from build123d import *

# Parameters (mm, degrees)
SKETCH_1_W               = 39
SKETCH_1_H               = 49
EXTRUDE_1_DEPTH          = 25
SKETCH_3_W               = 29
SKETCH_3_H               = 45
CUT_EXTRUDE_1_DEPTH      = 25
SKETCH_5_W               = 39
SKETCH_5_H               = 5
CUT_EXTRUDE_3_DEPTH      = 1
CUT_EXTRUDE_3_DEPTH_BACK = 26
HOLE_WIZARD_M4_4_D       = 3.3
SKETCH_20_W              = 39
SKETCH_20_H              = 5.65
CUT_EXTRUDE_5_DEPTH      = 1
CUT_EXTRUDE_5_DEPTH_BACK = 26
SKETCH_7_R               = 2.025
CUT_EXTRUDE_7_DEPTH      = 10
FILLET_1_R               = 2
FILLET_2_R               = 1
SKETCH_21_R              = 1.525
CUT_EXTRUDE_8_DEPTH      = 10


with BuildPart() as part:
    # 草图1 → 凸台-拉伸1 (new body)
    with BuildSketch(Plane.XY):
        Rectangle(SKETCH_1_W, SKETCH_1_H)
    extrude(amount=EXTRUDE_1_DEPTH)

    # 草图3 → 切除-拉伸1 (cut)
    with BuildSketch(Plane.XY.offset(25)):
        with Locations((0, -2)):
            Rectangle(SKETCH_3_W, SKETCH_3_H)
    extrude(amount=-CUT_EXTRUDE_1_DEPTH, mode=Mode.SUBTRACT)

    # 草图5 → 切除-拉伸3 (cut, two sides)
    with BuildSketch(Plane.XY.offset(25)) as cut_extrude_3_sk:
        with Locations((0, -22)):
            Rectangle(SKETCH_5_W, SKETCH_5_H)
    extrude(amount=CUT_EXTRUDE_3_DEPTH, mode=Mode.SUBTRACT)
    extrude(cut_extrude_3_sk.sketch, amount=-CUT_EXTRUDE_3_DEPTH_BACK, mode=Mode.SUBTRACT)

    # M4 螺纹孔4 (through all)
    with Locations(Plane(origin=(-19.5, 8.65, 5), x_dir=(0, 0, -1), z_dir=(-1, 0, 0))):
        with Locations((0, 0), (-15, 0), (-15, 15), (0, 15)):
            Hole(HOLE_WIZARD_M4_4_D / 2)

    # 草图20 → 切除-拉伸5 (cut, two sides)
    with BuildSketch(Plane.XY.offset(25)) as cut_extrude_5_sk:
        with Locations((0, -16.675)):
            Rectangle(SKETCH_20_W, SKETCH_20_H)
    extrude(amount=CUT_EXTRUDE_5_DEPTH, mode=Mode.SUBTRACT)
    extrude(cut_extrude_5_sk.sketch, amount=-CUT_EXTRUDE_5_DEPTH_BACK, mode=Mode.SUBTRACT)

    # 草图7 → 切除-拉伸7 (cut)
    with BuildSketch(Plane.XZ.offset(-20.5)):
        with Locations((-8.5, 20)):
            Circle(SKETCH_7_R)
        with Locations((-8.5, 5)):
            Circle(SKETCH_7_R)
        with Locations((8.5, 5)):
            Circle(SKETCH_7_R)
        with Locations((8.5, 20)):
            Circle(SKETCH_7_R)
    extrude(amount=-CUT_EXTRUDE_7_DEPTH, mode=Mode.SUBTRACT)

    # 圆角1
    fillet_1_edges = [part.edges().sort_by_distance(p)[0] for p in [
        (-14.5, 20.5, 12.5),
        (14.5, 20.5, 12.5),
        (-19.5, 24.5, 12.5),
        (19.5, 24.5, 12.5),
    ]]
    fillet(fillet_1_edges, radius=FILLET_1_R)

    # 圆角2
    fillet_2_edges = [part.edges().sort_by_distance(p)[0] for p in [
        (14.5, -13.85, 12.5),
        (-14.5, -13.85, 12.5),
        (-19.5, -13.85, 12.5),
        (19.5, -13.85, 12.5),
    ]]
    fillet(fillet_2_edges, radius=FILLET_2_R)

    # 草图21 → 切除-拉伸8 (cut)
    with BuildSketch(Plane(origin=(0, 24.5, 0), x_dir=(1, 0, 0), z_dir=(0, 1, 0))):
        with Locations((0, -6.15)):
            Circle(SKETCH_21_R)
        with Locations((0, -18.85)):
            Circle(SKETCH_21_R)
    extrude(amount=-CUT_EXTRUDE_8_DEPTH, mode=Mode.SUBTRACT)


solid = part.part
Read the model definition and answer for the solid it produces. Units are mm, in the model's axes. A direction names the side the tool comes from. Coordinates: 2 decimals unless noted, no trailing zeros. Loops run counter-clockwise (first coordinate to the right, second up) from the corner with the lowest first, then second, coordinate; pieces in that order, holes last. Notation, with made-up numbers: (49.5, 53) -> (54.5, 53) arc R11 ccw to (54.5, 74) -> close; hole circle Ø2 at (-27, -16). An arc over 180 degrees is marked (long way). Write item = value, one per line. Start each with the question number.
1) The part is cut by section B-B, the plane x = -8.5. Determine the outline of the cut face in (y, z) (3 decimals).
2) The part is cut by section A-A, the plane y = 13.5. Determine the outline of the cut face in (x, z), plus the area to 3 significant figures.
3) For faces 3 (the face through (17.03, -5.35, 18.69)), 4 (the face through (-14.5, 3, 13)), determine the directions among +Z, -Z, +X, -X, +Y, -Y from which every point of the face is accessible in a straight line to the end or side of a thin tool.
4) The part is cut by section D-D, the plane z = 16.5. Determine the outline of the cut face in (x, y).
5) The mould has two halves that part along X. Classify faces 1 (the face through (-16.97, -5.35, 3.69)), 2 (the face through (-0.2, 22.53, 17.34)): pulls with the +X half, pulls with the -X half, needs draft (parallel to the pull), parting line crosses it, or undercut.
6) Find the intervals of material crossed by L1, parallel to Z at x = 17.65, y = -6.35; L2, parallel to Z at x = 0, y = 22 (3 decimals); L3, parallel to Y at x = 16.9, z = 20, in increasing order. Write a range as from..to.
7) Given P1, Ø5.5, axis at x = -8.5, z = 20, coming from the -Y side, flat-ended and moving along its own axis, determine where the tip first touches the part or whether it passes through.
8) The part is cut by section C-C, the plane y = -6.35. Determine the outline of the cut face in (x, z), plus the area to 3 significant figures.
Result:
q1.outline = (20.5, 0) -> (24.5, 0) -> (24.5, 2.975) -> (20.5, 2.975) -> close; (20.5, 7.025) -> (24.5, 7.025) -> (24.5, 17.975) -> (20.5, 17.975) -> close; (20.5, 22.025) -> (24.5, 22.025) -> (24.5, 25) -> (20.5, 25) -> close
q2.outline = (-19.5, 0) -> (-14.5, 0) -> (-14.5, 25) -> (-19.5, 25) -> close; (14.5, 0) -> (19.5, 0) -> (19.5, 25) -> (14.5, 25) -> close
q2.area = 250 mm²
q3.face_3 = +X, -X
q3.face_4 = +Z, -Z, -Y
q4.outline = (-19.5, -12.85) arc R1 ccw to (-18.5, -13.85) -> (-15.5, -13.85) arc R1 ccw to (-14.5, -12.85) -> (-14.5, 18.5) arc R2 cw to (-12.5, 20.5) -> (12.5, 20.5) arc R2 cw to (14.5, 18.5) -> (14.5, -12.85) arc R1 ccw to (15.5, -13.85) -> (18.5, -13.85) arc R1 ccw to (19.5, -12.85) -> (19.5, 22.5) arc R2 ccw to (17.5, 24.5) -> (-17.5, 24.5) arc R2 ccw to (-19.5, 22.5) -> close
q5.face_1 = needs draft
q5.face_2 = undercut
q6.L1 = 0..3.35, 6.65..18.35, 21.65..25
q6.L2 = 0..4.625, 7.675..17.325, 20.375..25
q6.L3 = -13.85..-8, -4.7..7, 10.3..24.5
q7.P1 = 20.5
q8.outline = (-19.5, 0) -> (-14.5, 0) -> (-14.5, 3.35) -> (-19.5, 3.35) -> close; (-19.5, 6.65) -> (-14.5, 6.65) -> (-14.5, 18.35) -> (-19.5, 18.35) -> close; (-19.5, 21.65) -> (-14.5, 21.65) -> (-14.5, 25) -> (-19.5, 25) -> close; (14.5, 0) -> (19.5, 0) -> (19.5, 3.35) -> (14.5, 3.35) -> close; (14.5, 6.65) -> (19.5, 6.65) -> (19.5, 18.35) -> (14.5, 18.35) -> close; (14.5, 21.65) -> (19.5, 21.65) -> (19.5, 25) -> (14.5, 25) -> close
q8.area = 184 mm²
